Build history of the part. All positions in model axes, mm. A direction names the side the tool comes from. Round coordinates to 2 decimals unless told otherwise and drop trailing zeros. Loops run counter-clockwise (first coordinate to the right, second up) from the corner with the lowest first, then second, coordinate; pieces in that order, holes last. Notation, with made-up numbers: (85, 57) -> (104, 57) arc R30 cw to (104, 93) -> close; hole circle Ø7 at (75, -18). An arc over 180 degrees is marked (long way). Put each result on its own line as item: value. Start each with the question number.
Item 1: Tool access for faces 1 (the flat face through (17.5, 33, 20)), 2 (the flat face through (26, 48, 24)), 3 (the flat face through (7, 24, 25)), 4 (the flat face through (20, 25, 0)), 5 (the cylindrical face through (8, 32, 13)): list every direction of +Z, -Z, +X, -X, +Y, -Y with a clear straight run to the whole face (end or side of a thin tool).
Item 2: Pull direction X, two halves, no side cores. Call faces 6 (the flat face through (10, 0, 10)), 7 (the flat face through (8, 3, 20)), 8 (the flat face through (8, 30, 1)), 9 (the cylindrical face through (24.4, 43.9, 22.8)): +X half, -X half, draft (parallel to the pull), parting line (faces both ways), or undercut.
Item 3: Cut at C-C, the plane x = 13.5. List the corners of the cut face in (y, z), plus the area to 3 significant figures.
Item 4: Cut at A-A, the plane z = 24. List the corners of the cut face in (x, y).
Item 5: Cut at B-B, the plane y = 30. List the corners of the cut face in (x, z), plus the area to 3 significant figures.
Item 6: Flat gauge pins, fed straight in: pin 1 Ø2 at (y, z) = (4, 20) entering from +X; pin 2 Ø10 at (x, y) = (29, 19.5) entering from +Z; pin 3 Ø4.5 at (x, z) = (26, 24) entering from -Y; pin 4 Ø6 at (x, z) = (10.5, 21) entering from -Y. Where does each tip first touch, or does it go through?
Item 7: Drill centre lines: probe 1 along Z at (x, y) = (26, 42.25); probe 2 along X at (y, z) = (30, 15.5); probe 3 along Z at (x, y) = (31.5, 15). Where is each one in solid material? Low to high. Write a range as [from, to].
Item 8: Cut at D-D, the plane y = 44. List the corners of the cut face in (x, z), plus the area to 3 significant figures.
Autodesk Fusion 360 part; units mm, degrees
sketch "Sketch1" plane through (0, 0, 0) normal (0, 0, 1) x (1, 0, 0)
  line L0 (0, 0) -> (0, 50)
  line L1 (0, 0) -> (25, 0)
  line L2 (25, 0) -> (41.383, 11.4715)
  line L3 (25, 0) -> (45, 0) construction
  line L4 (0, 50) -> (41.383, 50)
  line L5 (41.383, 50) -> (41.383, 11.4715)
  dimension "d1" = 50
  dimension "d2" = 25
  dimension "d3" = 35
  dimension "d4" = 20
extrude "Extrude1" add sketch "Sketch1" along normal blind 40
extrude "Extrude2" cut 1 faces at (27.5887, 37.1572, 40) along direction (0, 0, -1) blind 25
sketch "Sketch2" plane through (0, 0, 15) normal (0, 0, 1) x (-1, 0, 0)
  line L0 (0, 0) -> (-25, 0)
  line L1 (-25, 0) -> (-41.383, -11.4715)
  line L2 (-41.383, -11.4715) -> (-41.383, -50)
  line L3 (-41.383, -50) -> (0, -50)
  line L4 (0, -50) -> (0, 0)
  line L5 (0, -40) -> (-30, -40)
  line L6 (0, 0) -> (-8, 0)
  line L7 (-8, -15) -> (-8, 0)
  line L8 (-15, -40) -> (-15, -30)
  line L9 (-8, -15) -> (-15, -30)
  line L10 (-30, -40) -> (-35, -40)
  line L11 (-35, -40) -> (-41.383, -47.2262)
extrude "Extrude3" add sketch "Sketch2" along normal blind 20 contours L2 L3 L4 L5 L10 L11
sketch "Sketch3" plane through (0, 0, 15) normal (0, 0, 1) x (-1, 0, 0)
  line L0 (-41.383, -47.2262) -> (-35, -40)
  line L1 (-35, -40) -> (0, -40)
  line L2 (0, -40) -> (0, 0)
  line L3 (0, 0) -> (-25, 0)
  line L4 (-25, 0) -> (-41.383, -11.4715)
  line L5 (-41.383, -11.4715) -> (-41.383, -47.2262)
  line L6 (-17.5, -40) -> (-17.5, -30)
  line L7 (-8, 0) -> (-8, -7)
  line L8 (-17.5, -30) -> (-17.5, -26)
  line L9 (-8, -7) -> (-17.5, -26)
extrude "Extrude4" add sketch "Sketch3" along normal blind 10 contours L1 L2 L3 L6 L7 L8 L9
sketch "Sketch4" plane through (0, 0, 25) normal (0, 0, 1) x (-1, 0, 0)
  line L0 (-17.5, -40) -> (0, -40)
  line L1 (0, -40) -> (0, 0)
  line L2 (0, 0) -> (-8, 0)
  line L3 (-8, 0) -> (-8, -7)
  line L4 (-8, -7) -> (-17.5, -26)
  line L5 (-17.5, -26) -> (-17.5, -40)
  circle A0 centre (-8, -30) radius 2
extrude "Extrude5" cut sketch "Sketch4" against normal blind 24 contours A0
sketch "Sketch5" plane through (0, 40, 0) normal (0, -1, 0) x (1, 0, 0)
  line L0 (17.5, 25) -> (17.5, 15)
  line L1 (17.5, 15) -> (35, 15)
  line L2 (35, 15) -> (35, 35)
  line L3 (35, 35) -> (0, 35)
  line L4 (0, 35) -> (0, 25)
  line L5 (0, 25) -> (17.5, 25)
sketch "Sketch6" plane through (0, 0, 25) normal (0, 0, 1) x (-1, 0, 0)
  circle A0 centre (-8, -30) radius 2
  line L0 (-17.5, -40) -> (0, -40)
  line L1 (0, -40) -> (0, 0)
  line L2 (0, 0) -> (-8, 0)
  line L3 (-8, 0) -> (-8, -7)
  line L4 (-8, -7) -> (-17.5, -26)
  line L5 (-17.5, -26) -> (-17.5, -40)
sketch "Sketch7" plane through (0, 40, 0) normal (0, -1, 0) x (1, 0, 0)
  circle A0 centre (26, 24) radius 2
  dimension "d17" = 4
extrude "Extrude6" cut sketch "Sketch7" against normal blind 8
Reply:
1. face 1: +Z, +X, -Y
1. face 2: -Y
1. face 3: +Z, +X, -X, -Y
1. face 4: -Z, +X, -X, +Y, -Y
1. face 5: +Z
2. face 6: draft
2. face 7: +X half
2. face 8: undercut
2. face 9: undercut
3. outline: (0, 0) -> (50, 0) -> (50, 35) -> (40, 35) -> (40, 25) -> (18, 25) -> (18, 15) -> (0, 15) -> close
3. area: 1,170 mm^2
4. outline: (0, 0) -> (8, 0) -> (8, 7) -> (17.5, 26) -> (17.5, 40) -> (24, 40) -> (24, 48) -> (28, 48) -> (28, 40) -> (35, 40) -> (41.38, 47.23) -> (41.38, 50) -> (0, 50) -> close; hole circle Ø4 at (8, 30)
5. outline: (0, 0) -> (41.38, 0) -> (41.38, 15) -> (17.5, 15) -> (17.5, 25) -> (10, 25) -> (10, 1) -> (6, 1) -> (6, 25) -> (0, 25) -> close
5. area: 700 mm^2
6. pin 1: stops at x = 8
6. pin 2: stops at z = 15
6. pin 3: stops at y = 40
6. pin 4: stops at y = 0
7. probe 1: z = [0, 22], [26, 35]
7. probe 2: x = [0, 6], [10, 17.5]
7. probe 3: z = [0, 15]
8. outline: (0, 0) -> (41.38, 0) -> (41.38, 15) -> (38.53, 15) -> (38.53, 35) -> (0, 35) -> close; hole circle Ø4 at (26, 24)
8. area: 1,380 mm^2
